```python
from build123d import *

# Parameters (mm, degrees)
F0_W      = 220
F0_H      = 40
F0_R      = 1.6
F1_DEPTH  = 1.5748
F2_W      = 10
F2_H      = 23
F3_DEPTH  = 17
F3_FACE_W = 10
F3_FACE_H = 17
F4_DEPTH  = 20
F5_R      = 2.5
F6_DEPTH  = 6.35


with BuildPart() as f1:
    # F0 (on Top) → F1 (new body)
    with BuildSketch(Plane.XY):
        Rectangle(F0_W, F0_H)
        with Locations((-106, -16)):
            Circle(F0_R, mode=Mode.SUBTRACT)
        with Locations((106, -16)):
            Circle(F0_R, mode=Mode.SUBTRACT)
        with Locations((-106, 16)):
            Circle(F0_R, mode=Mode.SUBTRACT)
        with Locations((106, 16)):
            Circle(F0_R, mode=Mode.SUBTRACT)
    extrude(amount=F1_DEPTH)

    # F2 (on face) → F3 (join)
    with BuildSketch(Plane(origin=(0, 0, 0), x_dir=(1, 0, 0), z_dir=(0, 0, -1))):
        with Locations((94, -8)):
            Rectangle(F2_W, F2_H)
    extrude(amount=F3_DEPTH)

    # F3_face (on face) → F4 (join)
    with BuildSketch(Plane(origin=(94, 19.5, -8.5), x_dir=(-1, 0, 0), z_dir=(0, 1, 0))):
        Rectangle(F3_FACE_W, F3_FACE_H)
    extrude(amount=F4_DEPTH)

    # F5 (on face) → F6 (join)
    with BuildSketch(Plane.XY.offset(1.5748)):
        with Locations((93, -11)):
            Circle(F5_R)
        with Locations((-96, -7)):
            Circle(F5_R)
        with Locations((74.5, 13)):
            Circle(F5_R)
    extrude(amount=F6_DEPTH)


solid = f1.part
```
Model file for the job. Use its own axes, mm. A direction names the side the tool comes from. Give positions to 0.01 mm unless a question says otherwise; leave off trailing zeros. Order: outer loops, then holes, each group sorted by start corner. A loop starts at its lowest first (then second) coordinate and runs counter-clockwise, first axis right, second up.
1) Saw through at B-B, the plane z = 3.5. Write the cut outline in (x, y).
2) Mould opens along X. For faces 1 (the cylindrical face through (73, 11, 5)), 2 (the flat face through (93, -11, 7.925)), 3 (the cylindrical face through (91, -12.5, 4.7)) say: +X half, -X half, draft (parallel to the pull), parting line (faces both ways), or undercut.
3) Wall check: probe 1 along Y at (x, z) = (-106, 1.3); probe 2 along X at (y, z) = (9, -14); probe 3 along Z at (x, y) = (24, -16). Give the ranges that are in metal, low to high.
4) Saw through at D-D, the plane z = -11.75. Write the cut outline in (x, y), then the cut area to 3 significant figures.
5) 3-axis set-ups, long thin cutter, end or side, ignore diameter. For faces 4 (the cylindrical face through (-98, -8.5, 4.7)), 5 (the flat face through (99, 18, -9)), 6 (the flat face through (94, -3.5, -8)), 7 (the flat face through (89, 18, -9)), 8 (the flat face through (94, 30, 0)): which of +Z, -Z, +X, -X, +Y, -Y reach the whole face in a straight line?
6) Saw through at A-A, the plane x = 74.5. Write the cut outline in (y, z).
7) Saw through at C-C, the plane y = 23.5. Write the cut outline in (x, z).
8) Pin check, flat tips, straight feed: pin 1 (8 mm diameter, centred on y = 30.5, z = -4, fed in from +X); pin 2 (8 mm diameter, centred on x = 53.5, z = 5, fed in from +Y); pin 3 (3 mm diameter, centred on x = 72, y = 8, fed in from -Z); pin 4 (8 mm diameter, centred on x = -7, z = 3.5, fed in from -Y). Stop position of each tip, or through.
Computed:
1. outline: circle Ø5 at (-96, -7); circle Ø5 at (74.5, 13); circle Ø5 at (93, -11)
2. face 1: parting line
2. face 2: draft
2. face 3: undercut
3. probe 1: y = -20 to -17.6, -14.4 to 14.4, 17.6 to 20
3. probe 2: x = 89 to 99
3. probe 3: z = 0 to 1.57
4. outline: (89, -3.5) - (99, -3.5) - (99, 39.5) - (89, 39.5) - close
4. area: 430 mm2
5. face 4: +Z
5. face 5: -Z, +X, +Y, -Y
5. face 6: -Z, +X, -X, -Y
5. face 7: -Z, -X, +Y, -Y
5. face 8: +Z, +X, -X, +Y
6. outline: (-20, 0) - (20, 0) - (20, 1.57) - (15.5, 1.57) - (15.5, 7.92) - (10.5, 7.92) - (10.5, 1.57) - (-20, 1.57) - close
7. outline: (89, -17) - (99, -17) - (99, 0) - (89, 0) - close
8. pin 1: stops at x = 99
8. pin 2: stops at y = 20
8. pin 3: stops at z = 0
8. pin 4: stops at y = -20
